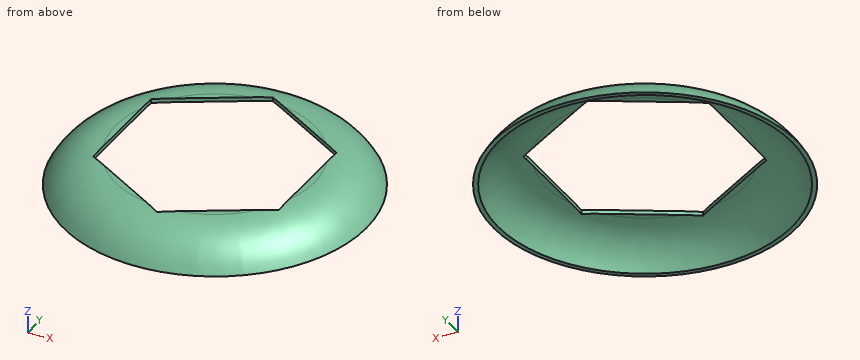
from build123d import *

# Parameters (mm, degrees)
F0_R     = 38.5
F1_DEPTH = 8
F4_DEPTH = 8
F5_T     = -1
F7_DEPTH = 25


# Not quite as in the source:
# - a fillet or chamfer that OpenCascade refuses, or shapes differently, is made with other operations: its cross-section is extruded or revolved along the edge and cut away or added


with BuildPart() as f1:
    # F0 (on Top) → F1 (new body)
    with BuildSketch(Plane.XY):
        Circle(F0_R)
    extrude(amount=F1_DEPTH)

    # F3: fillet of radius 15 on 1 edges, made by hand

    # F3_s1 → F3_t2 (revolve, cut)
    with BuildSketch(Plane.XZ):
        with BuildLine():
            ThreePointArc((38.5, 0), (32.979467531, 5.8452325787), (25.2335008386, 8))
            Line((25.2335008386, 8), (25.2335008386, 8.3))
            Line((25.2335008386, 8.3), (38.5, 8.3))
            Line((38.5, 8.3), (38.8, 8))
            ThreePointArc((38.8, 8), (38.8, 4), (38.7653299832, 0.14))
            Line((38.7653299832, 0.14), (38.5, 0))
        make_face()
    revolve(axis=Axis((0, 0, 8), (0, 0, 1)), mode=Mode.SUBTRACT)

    # F2 (on face) → F4 (cut)
    with BuildSketch(Plane.XY.offset(8)):
        Polygon((-0.0532552026, 25.9807075324), (-22.5265803327, 12.9442334078), (-22.47332513, -13.0364741246), (0.0532552026, -25.9807075324), (22.5265803327, -12.9442334078), (22.47332513, 13.0364741246), align=None)
    extrude(amount=-F4_DEPTH, mode=Mode.SUBTRACT)

    # F5
    f5_openings = [f1.faces().sort_by_distance(p)[0] for p in [
        (-37.411056, 0, 0),
    ]]
    offset(amount=F5_T, openings=f5_openings)

    # F6 (on Top) → F7 (cut)
    with BuildSketch(Plane.XY):
        Polygon((-23.56934, 13.6077647936), (-23.56934, -13.6077647936), (0, -27.2155295872), (23.56934, -13.6077647936), (23.56934, 13.6077647936), (0, 27.2155295872), align=None)
    extrude(amount=F7_DEPTH, mode=Mode.SUBTRACT)


solid = f1.part
The listing builds one solid part. Answer for the finished solid, in the listing's coordinates (mm). Give positions to 0.01 mm unless a question says otherwise; leave off trailing zeros. Loops run counter-clockwise (first coordinate to the right, second up) from the corner with the lowest first, then second, coordinate; pieces in that order, holes last. Notation, with made-up numbers: (-38, -6) - (7, -6) arc R22 ccw to (7, 32) - close; hole circle Ø8 at (-9, 5.5). An arc over 180 degrees is marked (long way). Answer as a JSON object with one key per item and string values.
1. Find the intervals of material crossed by L1, parallel to X at y = -11, z = 0.5; L2, parallel to Y at x = -25, z = 3; L3, parallel to Y at x = -6.5, z = 1.75, in increasing order. Write a range as [from, to].
Determined:
{"L1": "[-36.61, -35.38], [35.38, 36.61]", "L2": "[-26.48, -24.54], [24.54, 26.48]", "L3": "[-36.85, -35.57], [35.57, 36.85]"}
2. A cutting plane is placed at A-A (z = 2.25). Write down the section's boundary in (x, y).
Determined:
{"outline": "circle Ø74.08 at (0, 0); hole circle Ø71.48 at (0, 0)"}
3. Flat-ended cylindrical pins translate along their axes: pin 1 Ø3 at (y, z) = (21, 3) entering from +X; pin 2 Ø0.5 at (x, y) = (24.5, -0.5) entering from -Z; pin 3 Ø1 at (x, z) = (-16.5, 4) entering from -Y. Find the tip coordinate at first contact, or state that the pin passes through.
Determined:
{"pin 1": "x = 31.52", "pin 2": "z = 7", "pin 3": "y = -31.99"}
